Design review of the part built by this model. Coordinates are the model's own, in mm. A direction names the side the tool comes from. Coordinates: 2 decimals unless noted, no trailing zeros. Loops run counter-clockwise (first coordinate to the right, second up) from the corner with the lowest first, then second, coordinate; pieces in that order, holes last. Notation, with made-up numbers: (15.25, 24.25) -> (21.25, 24.25) arc R18 cw to (21.25, 33.25) -> close; hole circle Ø3 at (43.5, 77). An arc over 180 degrees is marked (long way). One line per item, written item: value. Start each with the question number.
1. Insertion check: pin 1 (2.5 mm diameter, centred on x = -71.5, z = 3.5, fed in from -Y); pin 2 (2.5 mm diameter, centred on y = 77, z = 3, fed in from +X); pin 3 (1.5 mm diameter, centred on x = -144, z = 2.5, fed in from +Y). Each pin has a flat end and moves straight along its axis. Give the tip position at first contact, or say it passes through.
2. Add section D-D on x = -30. Write out the cut boundary in (y, z).
3. Add section C-C on y = 61. Write out the cut boundary in (x, z), plus the area to 3 significant figures.
4. Draft analysis for pull direction Y (two halves, no side actions). For faces 6 (the flat face through (58, 20, 2)), 7 (the flat face through (145, 30, 2)), 8 (the flat face through (1.25, 27, 2)), 9 (the flat face through (-140, 41.92, 2)), state which applies: pulls with the +Y half, pulls with the -Y half, needs draft (parallel to the pull), parting line crosses it, or undercut.
5. Add section A-A on y = 78. Give the number of separate pieces and of enclosed holes in the cut face, plus the area to 3 significant figures.
6. For probe 1 along X at (y, z) = (53, 3.95); probe 2 along X at (y, z) = (34.5, 2.2); probe 3 along X at (y, z) = (64, 2.3), list the stretches that pass through material, from the lowest coordinate up.
7. Machinability: for faces 1 (the flat face through (-20.179, 17, 2)), 2 (the flat face through (145, 51.34, 2)), 3 (the flat face through (-118.547, 83.055, 2.465)), 4 (the flat face through (-145, 30, 2)), 5 (the flat face through (-75.179, 65, 2)), which of the approach directions +Z, -Z, +X, -X, +Y, -Y give a long, thin tool a straight path to every point of the face, cutting with its end or side? Answer none if there is none.
```python
from build123d import *

# Parameters (mm, degrees)
ESTRUSIONE_ESTRUSIONE1_DEPTH = 5
TAGLIO_ESTRUSIONE2_DEPTH     = 6
SCHIZZO5_W                   = 15
SCHIZZO5_H                   = 5
SCHIZZO5_W_2                 = 5
SCHIZZO5_H_2                 = 42.5
SCHIZZO5_W_3                 = 150.358983848
SCHIZZO5_H_3                 = 70
TAGLIO_ESTRUSIONE3_DEPTH     = 6
TAGLIO_ESTRUSIONE4_DEPTH     = 6
SCHIZZO7_R                   = 0.25
TAGLIO_ESTRUSIONE5_DEPTH     = 10


with BuildPart() as part:
    # Schizzo1 → Estrusione-Estrusione1 (new body)
    with BuildSketch(Plane.XY):
        Polygon((-142.5, 75), (-142.5, 66.339745962), (-147.5, 66.339745962), (-147.5, 51.339745962), (-142.5, 51.339745962), (-142.5, 30), (-147.5, 30), (-147.5, 15), (-142.5, 15), (-142.5, 0), (142.5, 0), (142.5, 15), (147.5, 15), (147.5, 30), (142.5, 30), (142.5, 51.339745962), (147.5, 51.339745962), (147.5, 66.339745962), (142.5, 66.339745962), (142.5, 75), (99.198729811, 100), (-99.198729811, 100), align=None)
    extrude(amount=ESTRUSIONE_ESTRUSIONE1_DEPTH)

    # Schizzo2 → Taglio-Estrusione2 (cut, through all)
    with BuildSketch(Plane.XY):
        Polygon((-99.198729811, 82.679491924), (-127.5, 66.339745962), (-127.5, 49.330127019), (-99.198729811, 65.669872981), align=None)
        Polygon((99.198729811, 31.339745962), (99.198729811, 48.349364905), (127.5, 32.009618943), (127.5, 15), align=None)
        Polygon((-95.179491924, 15), (-121.160254038, 0), (121.160254038, 0), (95.179491924, 15), align=None)
        Polygon((-99.198729811, 31.339745962), (-127.5, 15), (-127.5, 32.009618943), (-99.198729811, 48.349364905), align=None)
        Polygon((99.198729811, 65.669872981), (99.198729811, 82.679491924), (127.5, 66.339745962), (127.5, 49.330127019), align=None)
        Polygon((-132.5, 75), (-104.198729811, 91.339745962), (-101.698729811, 87.009618943), (-130, 70.669872981), align=None)
        Polygon((132.5, 75), (130, 70.669872981), (101.698729811, 87.009618943), (104.198729811, 91.339745962), align=None)
    extrude(amount=TAGLIO_ESTRUSIONE2_DEPTH, mode=Mode.SUBTRACT)

    # Schizzo5 → Taglio-Estrusione3 (cut, through all)
    with BuildSketch(Plane.XY):
        with Locations((-87.679491924, 17.5)):
            Rectangle(SCHIZZO5_W, SCHIZZO5_H)
        with Locations((-57.679491924, 17.5)):
            Rectangle(SCHIZZO5_W, SCHIZZO5_H)
        with Locations((-27.679491924, 17.5)):
            Rectangle(SCHIZZO5_W, SCHIZZO5_H)
        with Locations((27.679491924, 17.5)):
            Rectangle(SCHIZZO5_W, SCHIZZO5_H)
        with Locations((57.679491924, 17.5)):
            Rectangle(SCHIZZO5_W, SCHIZZO5_H)
        with Locations((87.679491924, 17.5)):
            Rectangle(SCHIZZO5_W, SCHIZZO5_H)
        with Locations((87.679491924, 78.75)):
            Rectangle(SCHIZZO5_W_2, SCHIZZO5_H_2)
        with Locations((-87.679491924, 78.75)):
            Rectangle(SCHIZZO5_W_2, SCHIZZO5_H_2)
        with Locations((0, 65)):
            Rectangle(SCHIZZO5_W_3, SCHIZZO5_H_3)
    extrude(amount=TAGLIO_ESTRUSIONE3_DEPTH, mode=Mode.SUBTRACT)

    # Schizzo6 → Taglio-Estrusione4 (cut, through all)
    with BuildSketch(Plane.XY):
        Polygon((-142.5, 41.919872981), (-136.5, 41.919872981), (-136.5, 43.419872981), (-134.1, 43.419872981), (-134.1, 41.919872981), (-132.5, 41.919872981), (-132.5, 39.419872981), (-134.1, 39.419872981), (-134.1, 37.919872981), (-136.5, 37.919872981), (-136.5, 39.419872981), (-142.5, 39.419872981), align=None)
        Polygon((134.1, 43.419872981), (134.1, 41.919872981), (132.5, 41.919872981), (132.5, 39.419872981), (134.1, 39.419872981), (134.1, 37.919872981), (136.5, 37.919872981), (136.5, 39.419872981), (142.5, 39.419872981), (142.5, 41.919872981), (136.5, 41.919872981), (136.5, 43.419872981), align=None)
        Polygon((-88.929491924, 20), (-88.929491924, 26), (-90.429491924, 26), (-90.429491924, 28.4), (-88.929491924, 28.4), (-88.929491924, 30), (-86.429491924, 30), (-86.429491924, 28.4), (-84.929491924, 28.4), (-84.929491924, 26), (-86.429491924, 26), (-86.429491924, 20), align=None)
        Polygon((86.429491924, 20), (88.929491924, 20), (88.929491924, 26), (90.429491924, 26), (90.429491924, 28.4), (88.929491924, 28.4), (88.929491924, 30), (86.429491924, 30), (86.429491924, 28.4), (84.929491924, 28.4), (84.929491924, 26), (86.429491924, 26), align=None)
        Polygon((-1.25, 20), (-1.25, 21.6), (-2.75, 21.6), (-2.75, 24), (-1.25, 24), (-1.25, 30), (1.25, 30), (1.25, 24), (2.75, 24), (2.75, 21.6), (1.25, 21.6), (1.25, 20), align=None)
    extrude(amount=TAGLIO_ESTRUSIONE4_DEPTH, mode=Mode.SUBTRACT)

    # Schizzo7 → Taglio-Estrusione5 (cut)
    with BuildSketch(Plane.XY.offset(5)):
        with Locations((-136.5, 43.419872981)):
            Circle(SCHIZZO7_R)
        with Locations((-136.5, 37.919872981)):
            Circle(SCHIZZO7_R)
        with Locations((-90.429491924, 26)):
            Circle(SCHIZZO7_R)
        with Locations((-84.929491924, 26)):
            Circle(SCHIZZO7_R)
        with Locations((-2.75, 24)):
            Circle(SCHIZZO7_R)
        with Locations((2.75, 24)):
            Circle(SCHIZZO7_R)
        with Locations((84.929491924, 26)):
            Circle(SCHIZZO7_R)
        with Locations((90.429491924, 26)):
            Circle(SCHIZZO7_R)
        with Locations((136.5, 43.419872981)):
            Circle(SCHIZZO7_R)
        with Locations((136.5, 37.919872981)):
            Circle(SCHIZZO7_R)
    extrude(amount=-TAGLIO_ESTRUSIONE5_DEPTH, mode=Mode.SUBTRACT)


solid = part.part
```
Worked answers:
1. pin 1: stops at y = 15
1. pin 2: stops at x = 141.2
1. pin 3: stops at y = 66.34
2. outline: (20, 0) -> (30, 0) -> (30, 5) -> (20, 5) -> close
3. outline: (-147.5, 0) -> (-127.5, 0) -> (-127.5, 5) -> (-147.5, 5) -> close; (-107.29, 0) -> (-90.18, 0) -> (-90.18, 5) -> (-107.29, 5) -> close; (-85.18, 0) -> (-75.18, 0) -> (-75.18, 5) -> (-85.18, 5) -> close; (75.18, 0) -> (85.18, 0) -> (85.18, 5) -> (75.18, 5) -> close; (90.18, 0) -> (107.29, 0) -> (107.29, 5) -> (90.18, 5) -> close; (127.5, 0) -> (147.5, 0) -> (147.5, 5) -> (127.5, 5) -> close
3. area: 471 mm²
4. face 6: pulls with the -Y half
4. face 7: undercut
4. face 8: needs draft
4. face 9: undercut
5. separate pieces: 8
5. enclosed holes: 0
5. area: 390 mm²
6. probe 1: x = -147.5 to -127.5, -121.14 to -75.18, 75.18 to 121.14, 127.5 to 147.5
6. probe 2: x = -142.5 to -123.19, -99.2 to -75.18, 75.18 to 99.2, 123.19 to 142.5
6. probe 3: x = -147.5 to -127.5, -102.09 to -90.18, -85.18 to -75.18, 75.18 to 85.18, 90.18 to 102.09, 127.5 to 147.5
7. face 1: +Z, -Z, -Y
7. face 2: +Z, -Z, +X
7. face 3: +Z, -Z
7. face 4: +Z, -Z, -X
7. face 5: +Z, -Z, +Y
